```python
from build123d import *

# Parameters (mm, degrees)
SKETCH1_R             = 72.5
BOSS_EXTRUDE1_DEPTH   = 21
SKETCH2_R             = 15
CUT_EXTRUDE1_DEPTH    = 105.658969993
SKETCH3_R             = 7.570186168
CUT_EXTRUDE2_DEPTH    = 15.436386
CIRPATTERN1_START     = 5.563613899
CIRPATTERN1_OUTLINE_R = 7.570186168
CIRPATTERN1_DEPTH     = 15.436386101


# Read off the part's stored shape, not the designer's step: CirPattern1
with BuildPart() as part:
    # Sketch1 → Boss-Extrude1 (new body)
    with BuildSketch(Plane(origin=(0, 0, 0), x_dir=(1, 0, 0), z_dir=(0, 1, 0))):
        with Locations(Location((0, 0, 0), (0, 0, 90))):
            Circle(SKETCH1_R)
    extrude(amount=BOSS_EXTRUDE1_DEPTH)

    # Sketch2 → Cut-Extrude1 (cut, through all)
    with BuildSketch(Plane(origin=(0, 0, 0), x_dir=(1, 0, 0), z_dir=(0, 1, 0))):
        with Locations(Location((0, 0, 0), (0, 0, 90))):
            Circle(SKETCH2_R)
    extrude(amount=CUT_EXTRUDE1_DEPTH, mode=Mode.SUBTRACT)

    # Sketch3 → Cut-Extrude2 (cut)
    with BuildSketch(Plane(origin=(0, 21, 0), x_dir=(1, 0, 0), z_dir=(0, 1, 0))):
        with Locations(Location((-22.754654532, 0, 0), (0, 0, 270))):
            Circle(SKETCH3_R)
    extrude(amount=-CUT_EXTRUDE2_DEPTH, mode=Mode.SUBTRACT)

    # CirPattern1 outline → CirPattern1 (cut)
    with BuildSketch(Plane(origin=(0, 0, 0), x_dir=(1, 0, 0), z_dir=(0, 1, 0)).offset(CIRPATTERN1_START)):
        with Locations((0, 22.754654532)):
            Circle(CIRPATTERN1_OUTLINE_R)
        with Locations((22.754654532, 0)):
            Circle(CIRPATTERN1_OUTLINE_R)
        with Locations((0, -22.754654532)):
            Circle(CIRPATTERN1_OUTLINE_R)
    extrude(amount=CIRPATTERN1_DEPTH, mode=Mode.SUBTRACT)


solid = part.part
```
Design review of the part built by this model. Coordinates are the model's own, in mm. A direction names the side the tool comes from. Coordinates: 2 decimals unless noted, no trailing zeros. Order: outer loops, then holes, each group sorted by start corner. A loop starts at its lowest first (then second) coordinate and runs counter-clockwise, first axis right, second up. Notation, with made-up numbers: (34, 13) - (74, 13) arc R27 cw to (74, 33) - close; hole circle Ø6 at (57.25, -28.75). An arc over 180 degrees is marked (long way). One line per question, with ' | ' between items.
Q1. The part is to be moulded in two halves that separate along X. For faces 1 (the flat face through (-17, 0, 1)), 2 (the flat face through (0, 5.564, 23)), 3 (the cylindrical face through (-21.78, 10.35, -69.15)), say which applies: +X half, -X half, draft (parallel to the pull), parting line (faces both ways), or undercut.
Answer key:
face 1: draft | face 2: undercut | face 3: parting line
Q2. Consider section D-D, the plane z = -25. Give the boundary of the cut face in (x, y), then the cut area to 3 significant figures.
Answer key:
outline: (-68.05, 0) - (68.05, 0) - (68.05, 21) - (7.23, 21) - (7.23, 5.56) - (-7.23, 5.56) - (-7.23, 21) - (-68.05, 21) - close | area: 2,640 mm2
Q3. Clearance check with flat-ended pins moving along their axes: pin 1 Ø7.5 at (x, z) = (1, 22) entering from +Y; pin 2 Ø1.5 at (y, z) = (7.5, -41) entering from +X; pin 3 Ø24 at (x, z) = (0, 0) entering from +Y; pin 4 Ø2 at (y, z) = (12.5, -22) entering from +X. State where each tip first meets the part, or that it passes through.
Answer key:
pin 1: stops at y = 5.56 | pin 2: stops at x = 60.3 | pin 3: passes through | pin 4: stops at x = 69.39
Q4. Consider section A-A, the plane z = 0. Give the boundary of the cut face in (x, y), then the cut area to 3 significant figures.
Answer key:
outline: (-72.5, 0) - (-15, 0) - (-15, 21) - (-15.18, 21) - (-15.18, 5.56) - (-30.32, 5.56) - (-30.32, 21) - (-72.5, 21) - close; (15, 0) - (72.5, 0) - (72.5, 21) - (30.32, 21) - (30.32, 5.56) - (15.18, 5.56) - (15.18, 21) - (15, 21) - close | area: 1,950 mm2
Q5. Consider section B-B, the plane x = 0. Give the boundary of the cut face in (y, z).
Answer key:
outline: (0, -72.5) - (21, -72.5) - (21, -30.32) - (5.56, -30.32) - (5.56, -15.18) - (21, -15.18) - (21, -15) - (0, -15) - close; (0, 15) - (21, 15) - (21, 15.18) - (5.56, 15.18) - (5.56, 30.32) - (21, 30.32) - (21, 72.5) - (0, 72.5) - close
Q6. To check wall thickness, follow line 1 along X through (y, z) = (14.25, 0); line 2 along Z through (x, y) = (-5, 11); line 3 along X through (y, z) = (5, 0). State the ranges of each line that lie inside material, in increasing order.
Answer key:
line 1: x = -72.5 to -30.32, -15.18 to -15, 15 to 15.18, 30.32 to 72.5 | line 2: z = -72.33 to -28.44, -17.07 to -14.14, 14.14 to 17.07, 28.44 to 72.33 | line 3: x = -72.5 to -15, 15 to 72.5
Q7. Consider section C-C, the plane x = -27.5. Give the boundary of the cut face in (y, z), then the cut area to 3 significant figures.
Answer key:
outline: (0, -67.08) - (21, -67.08) - (21, -5.9) - (5.56, -5.9) - (5.56, 5.9) - (21, 5.9) - (21, 67.08) - (0, 67.08) - close | area: 2,640 mm2
Q8. For faces 4 (the flat face through (15, 21, -15)), 5 (the flat face through (23, 5.564, 0)), list the 3-axis set-ups (+Z, -Z, +X, -X, +Y, -Y) from which the entire face can be reached by the end or side of a thin tool; tool diameter is ignored.
Answer key:
face 4: +Z, -Z, +X, -X, +Y | face 5: +Y
